Design review of the part built by this model. Coordinates are the model's own, in mm. A direction names the side the tool comes from. Coordinates: 2 decimals unless noted, no trailing zeros. Loops run counter-clockwise (first coordinate to the right, second up) from the corner with the lowest first, then second, coordinate; pieces in that order, holes last. Notation, with made-up numbers: M 23,66 L 76,66 A28 cw 76,90 Z; hole C 69,-9.75 d1. An arc over 180 degrees is marked long. Write item = value, one per line. Start each with the question number.
```python
from build123d import *

# Parameters (mm, degrees)
F0_R     = 11
F1_DEPTH = 2
F2_R     = 5
F2_R_2   = 3.5
F3_DEPTH = 9
F4_R     = 3.5
F5_DEPTH = 2
F7_D     = 2.5
F10_D    = 2.5


with BuildPart() as f1:
    # F0 (on Top) → F1 (new body)
    with BuildSketch(Plane.XY):
        Circle(F0_R)
    extrude(amount=F1_DEPTH)

    # F2 (on face) → F3 (join)
    with BuildSketch(Plane.XY.offset(2)):
        Circle(F2_R)
        Circle(F2_R_2, mode=Mode.SUBTRACT)
    extrude(amount=F3_DEPTH)

    # F4 (on face) → F5 (cut, through all)
    with BuildSketch(Plane.XY.offset(2)):
        Circle(F4_R)
    extrude(amount=-F5_DEPTH, mode=Mode.SUBTRACT)

    # F7 (through all)
    with Locations(Plane.XY.offset(2)):
        with Locations((0, 8), (8, 0), (0, -8), (-8, 0)):
            Hole(F7_D / 2)

    # F10 (through all)
    with Locations(Plane.YZ.offset(5)):
        with Locations((0, 6.5)):
            Hole(F10_D / 2)


solid = f1.part
```
(1) Insertion check: pin 1 (3 mm diameter, centred on y = 0, z = 6.5, fed in from +X); pin 2 (11 mm diameter, centred on x = 0, y = 0, fed in from -Z); pin 3 (6 mm diameter, centred on x = 0, z = 8, fed in from +Y); pin 4 (1 mm diameter, centred on x = 7.5, z = 2, fed in from -Y). Each pin has a flat end and moves straight along its axis. Give the tip position at first contact, or say it passes through.
(2) Mouldability with a two-part tool opening along X and no side actions: class faces 3 (the cylindrical face through (4.77, 1.5, 6.44)), 4 (the cylindrical face through (0.27, 6.78, 0.99)), 5 (the flat face through (-3, 3, 0)) as +X half, -X half, draft (parallel to the pull), parting line (faces both ways), or undercut.
(3) Tool access review of faces 1 (the cylindrical face through (4.12, 0.27, 5.28)), 2 (the flat face through (5, -2, 2)): name each direction out of +Z, -Z, +X, -X, +Y, -Y from which nothing blocks a thin tool from reaching the whole face with its end or side.
(4) Take a section at B-B (y = 7.25). State the section outline as (x, z) points, plus the area to 3 significant figures.
(5) To check wall thickness, follow L1, parallel to Z at x = -5, y = 3; L2, parallel to Y at x = 0, z = 7.25; L3, parallel to X at y = -1.75, z = 10.5. State the ranges of each line that lie inside material, in increasing order.
(6) Take a section at D-D (y = 0.5). State the section outline as (x, z) points, plus the area to 3 significant figures.
(7) Take a section at A-A (x = 0). State the section outline as (y, z) points, plus the area to 3 significant figures.
Results list:
q1.pin_1 = 5
q1.pin_2 = 0
q1.pin_3 = 5
q1.pin_4 = -8.49
q2.face_3 = parting line
q2.face_4 = undercut
q2.face_5 = draft
q3.face_1 = +X, -X
q3.face_2 = +Z
q4.outline = M -8.27,0 L -1,0 L -1,2 L -8.27,2 Z; M 1,0 L 8.27,0 L 8.27,2 L 1,2 Z
q4.area = 29.1 mm^2
q5.L1 = 0 to 2
q5.L2 = -5 to -3.5, 3.5 to 5
q5.L3 = -4.68 to -3.03, 3.03 to 4.68
q6.outline = M -10.99,0 L -9.15,0 L -9.15,2 L -10.99,2 Z; M -6.85,0 L -3.46,0 L -3.46,5.35 L -4.97,5.35 L -4.97,2 L -6.85,2 Z; M -4.97,7.65 L -3.46,7.65 L -3.46,11 L -4.97,11 Z; M 3.46,0 L 6.85,0 L 6.85,2 L 4.97,2 L 4.97,5.35 L 3.46,5.35 Z; M 3.46,7.65 L 4.97,7.65 L 4.97,11 L 3.46,11 Z; M 9.15,0 L 10.99,0 L 10.99,2 L 9.15,2 Z
q6.area = 41.2 mm^2
q7.outline = M -11,0 L -9.25,0 L -9.25,2 L -11,2 Z; M -6.75,0 L -3.5,0 L -3.5,11 L -5,11 L -5,2 L -6.75,2 Z; M 3.5,0 L 6.75,0 L 6.75,2 L 5,2 L 5,11 L 3.5,11 Z; M 9.25,0 L 11,0 L 11,2 L 9.25,2 Z
q7.area = 47.0 mm^2
